```python
from build123d import *

# Parameters (mm, degrees)
SKETCH2_R           = 7.5
SKETCH1_R           = 27.5
SKETCH2_2_R         = 7.5
BOSS_EXTRUDE1_DEPTH = 162
SKETCH3_R           = 22.5
BOSS_EXTRUDE2_DEPTH = 5
CUT_EXTRUDE3_START  = -10
CUT_EXTRUDE3_DEPTH  = 10
SKETCH21_R          = 5
CUT_EXTRUDE4_DEPTH  = 20


with BuildPart() as part:
    # Sketch2 → Loft1 section 0
    with BuildSketch(Plane(origin=(0, 30, 0), x_dir=(1, 0, 0), z_dir=(0, 1, 0))):
        Circle(SKETCH2_R)
    # Sketch1 → Loft1 section 1
    with BuildSketch(Plane(origin=(0, 0, 0), x_dir=(1, 0, 0), z_dir=(0, 1, 0))):
        Circle(SKETCH1_R)
    loft()

    # Sketch2<2> → Boss-Extrude1 (add)
    with BuildSketch(Plane(origin=(0, 30, 0), x_dir=(1, 0, 0), z_dir=(0, 1, 0))):
        with Locations(Location((0, 0, 0), (0, 0, 90))):
            Circle(SKETCH2_2_R)
    extrude(amount=BOSS_EXTRUDE1_DEPTH)

    # Sketch3 → Boss-Extrude2 (add)
    with BuildSketch(Plane(origin=(0, 177, 0), x_dir=(1, 0, 0), z_dir=(0, 1, 0))):
        with Locations(Location((0, 0, 0), (0, 0, 270))):
            Circle(SKETCH3_R)
    extrude(amount=BOSS_EXTRUDE2_DEPTH)

    # Sketch5 → Cut-Extrude3 (cut)
    with BuildSketch(Plane(origin=(0, 192, 0), x_dir=(1, 0, 0), z_dir=(0, 1, 0)).offset(CUT_EXTRUDE3_START)):
        with BuildLine():
            ThreePointArc((7.5, 0), (6.123724357, 4.330127019), (2.5, 7.071067812))
            Line((2.5, 7.071067812), (2.5, -7.071067812))
            ThreePointArc((2.5, -7.071067812), (6.123724357, -4.330127019), (7.5, 0))
        make_face()
        with BuildLine():
            Line((-2.5, -7.071067812), (-2.5, 7.071067812))
            ThreePointArc((-2.5, 7.071067812), (-7.5, 0), (-2.5, -7.071067812))
        make_face()
    extrude(amount=CUT_EXTRUDE3_DEPTH, mode=Mode.SUBTRACT)

    # Sketch21 → Cut-Extrude4 (cut)
    with BuildSketch(Plane.XZ):
        with Locations(Location((0, 0, 0), (0, 0, 270))):
            Circle(SKETCH21_R)
    extrude(amount=-CUT_EXTRUDE4_DEPTH, mode=Mode.SUBTRACT)


solid = part.part
```
Geometry check sheet. Reference: the model listing, model coordinates, mm. A direction names the side the tool comes from. Give positions to 0.01 mm unless a question says otherwise; leave off trailing zeros. Order: outer loops, then holes, each group sorted by start corner. A loop starts at its lowest first (then second) coordinate and runs counter-clockwise, first axis right, second up. Notation, with made-up numbers: (-18.75, 26) - (0.25, 26) arc R17 ccw to (0.25, 38) - close; hole circle Ø1 at (29, 44.5). An arc over 180 degrees is marked (long way). Answer in a Markdown table with one row per item. Add a question column.
Q1. Material ranges on probe 1 along X at (y, z) = (7.5, 0); probe 2 along X at (y, z) = (4.75, 0); probe 3 along Y at (x, z) = (-5, 10.5), recorded low to high. Write a range as from..to.
Q2. Mould release check, pull along Y, two halves, no side actions. Record for faces 1 (the flat face through (0, 0, 6)), 2 (the cylindrical face through (-0.33, 102.471, 7.493)), 3 (the flat face through (0, 192, 0)): pulls with the +Y half, pulls with the -Y half, needs draft (parallel to the pull), parting line crosses it, or undercut.
Q3. Cross-section at A-A, the plane y = 116.5. Enter the section's corners in (x, z), then the cut area to 3 significant figures.
Q4. Cross-section at B-B, the plane y = 23. Enter the section's corners in (x, z).
Q5. Gauge pin test, flat ends, axial feed: pin 1 (8 mm diameter, centred on x = 0, z = 0, fed in from -Y); pin 2 (2 mm diameter, centred on x = -2, z = 10.5, fed in from +Y); pin 3 (10 mm diameter, centred on y = 64.5, z = -1.5, fed in from +X). Record the tip position at first contact, or that the pin passes through.
Q6. Tool access check on faces 4 (the cylindrical face through (0, 186.9, -7.5)), 5 (the conical face through (-2.86, 21.46, 12.88)), 6 (the flat face through (2.5, 187, 0)), 7 (the cylindrical face through (0, 186.9, 7.5)), 8 (the cylindrical face through (-4.88, 9.86, 1.08)). Record the directions out of +Z, -Z, +X, -X, +Y, -Y that give a thin tool (end or side, any length) a straight path to the whole face; none if there is none.
Check values:
| question | item | result |
|---|---|---|
| 1 | probe 1 | x = -22.5..-5, 5..22.5 |
| 1 | probe 2 | x = -24.33..-5, 5..24.33 |
| 1 | probe 3 | y = 0..23.81, 177..182 |
| 2 | face 1 | pulls with the -Y half |
| 2 | face 2 | undercut |
| 2 | face 3 | pulls with the +Y half |
| 3 | outline | circle Ø15 at (0, 0) |
| 3 | area | 177 mm^2 |
| 4 | outline | circle Ø24.33 at (0, 0) |
| 5 | pin 1 | stops at y = 20 |
| 5 | pin 2 | stops at y = 182 |
| 5 | pin 3 | stops at x = 7.5 |
| 6 | face 4 | -Z, +Y |
| 6 | face 5 | none |
| 6 | face 6 | +Z, -Z, +X, +Y |
| 6 | face 7 | +Z, +Y |
| 6 | face 8 | -Y |
